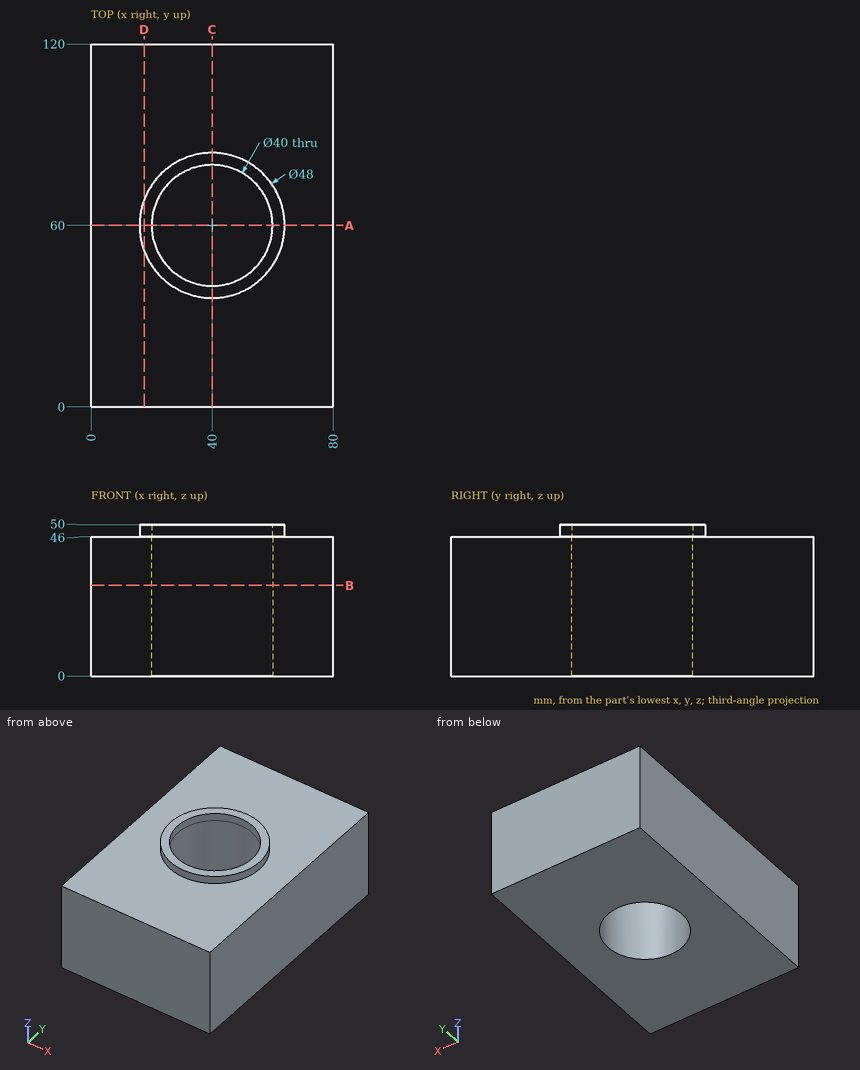
Could you check a few things on this drawing? It's one solid part, dimensions in mm from its lowest x, y, z. Coordinates: 2 decimals unless noted, no trailing zeros. Write each loop counter-clockwise with the first axis right and the second up, starting at its lowest first coordinate (ties: lowest second). Pieces come first, ordered by that corner, then holes.
Q1. Imagine slicing it at D-D, the plane x = 17.5. List the corners of the cut face in (y, z) for me.
Results found:
outline: (0, 0) - (120, 0) - (120, 46) - (68.35, 46) - (68.35, 50) - (51.65, 50) - (51.65, 46) - (0, 46) - close
Q2. For P1, Ø1, axis at y = 58.5, z = 27.5, coming from the -X side; P2, Ø1.5, axis at x = 14.5, y = 107.5, coming from the +Z side, each with a flat end and sliding along its axis, tell me the tip position at first contact or that it passes through.
Results found:
P1: stops at x = 0
P2: stops at z = 46
Q3. Imagine slicing it at C-C, the plane x = 40. List the corners of the cut face in (y, z) for me.
Results found:
outline: (0, 0) - (40, 0) - (40, 50) - (36, 50) - (36, 46) - (0, 46) - close; (80, 0) - (120, 0) - (120, 46) - (84, 46) - (84, 50) - (80, 50) - close
Q4. Imagine slicing it at B-B, the plane z = 30. List the corners of the cut face in (x, y) for me, plus the area to 3 significant figures.
Results found:
outline: (0, 0) - (80, 0) - (80, 120) - (0, 120) - close; hole circle Ø40 at (40, 60)
area: 8,340 mm2
Q5. Please list where these lines run through material, in increasing order: L1, parallel to Y at x = 40, z = 47.8; L2, parallel to Y at x = 40, z = 22; L3, parallel to X at y = 50.5, z = 6.5.
Results found:
L1: y = 36 to 40, 80 to 84
L2: y = 0 to 40, 80 to 120
L3: x = 0 to 22.4, 57.6 to 80
Q6. Imagine slicing it at A-A, the plane y = 60. List the corners of the cut face in (x, z) for me.
Results found:
outline: (0, 0) - (20, 0) - (20, 50) - (16, 50) - (16, 46) - (0, 46) - close; (60, 0) - (80, 0) - (80, 46) - (64, 46) - (64, 50) - (60, 50) - close
